Geometry check sheet. Reference: the model listing, model coordinates, mm. Face numbers are marked on the shaded views. Give positions to 0.01 mm unless a question says otherwise; leave off trailing zeros. Loops run counter-clockwise (first coordinate to the right, second up) from the corner with the lowest first, then second, coordinate; pieces in that order, holes last.
1. Release check for a two-part mould opening along Y. For the marked faces 1, 2 and 3 record: +Y half, -Y half, draft (parallel to the pull), parting line (faces both ways), or undercut.
2. Cross-section at A-A, the plane y = -6.5. Record the cut outline in (x, z), plus the area to 3 significant figures.
3. Material ranges on L1, parallel to Z at x = 0, y = -25.5; L2, parallel to Z at x = -4.25, y = 27.5; L3, parallel to X at y = 11, z = -1.5, recorded low to high.
4. Go/stop test with flat-tipped pins: pin 1 Ø1 at (x, z) = (4.5, 0.5) entering from +Y; pin 2 Ø1.5 at (x, y) = (-4, -6.5) entering from -Z; pin 3 Ø2 at (x, y) = (1, -8.5) entering from -Z. Record where each tip stops, or that it passes through.
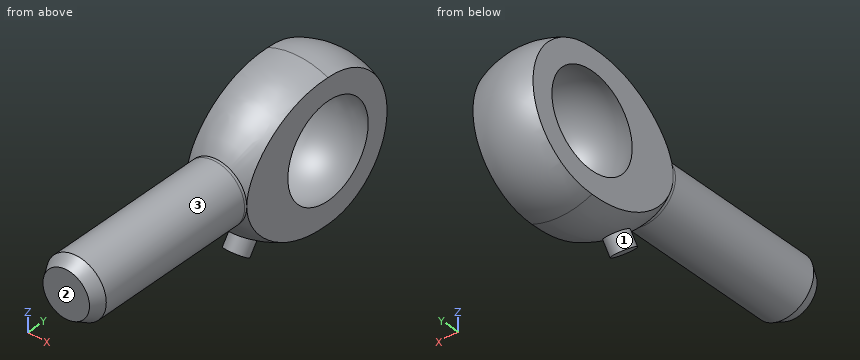
Autodesk Inventor part; units mm, degrees
ref_plane "IP1_XY" through (0, 21, 0) normal (1, 0, 0) x (0, 0, -1)
ref_plane "IP1_YZ" through (0, 21, 0) normal (0, 0, -1) x (0, 1, 0)
ref_plane "IP1_ZX" through (0, 21, 0) normal (0, 1, 0) x (1, 0, 0)
sketch "Sketch_5" plane through (0, 0, 0) normal (0, 0, 1) x (1, 0, 0)
  line L0 (0, -33) -> (0, 36)
  arc A0 (15, 21) -> (0, 36) centre (0, 21) ccw
  arc A1 (6, 2.0892) -> (15, 21) centre (-7.4821, 20.1026) ccw
  arc A2 (6, 2.0892) -> (6, 1.56) centre (8.9883, 1.8246) ccw
  line L1 (6, 1.56) -> (6, -30.66)
  line L2 (6, -30.66) -> (4.649, -33)
  line L3 (4.649, -33) -> (0, -33)
  line L4 (0, -33) -> (0, 36)
revolve "Revolution1" add sketch "Sketch_5" angle 360 about axis through (0, -33, 0) along (0, -1, 0)
thread "Thread1"
sketch "Sketch_6" plane through (0, 0, 0) normal (0, 0, 1) x (1, 0, 0)
  line L0 (-22.5, 37.8) -> (-22.5, -34.65)
  line L1 (-22.5, -34.65) -> (22.5, -34.65)
  line L2 (22.5, -34.65) -> (22.5, 37.8)
  line L3 (22.5, 37.8) -> (-22.5, 37.8)
  line L4 (-6, 36) -> (-6, -33)
  line L5 (-6, -33) -> (6, -33)
  line L6 (6, -33) -> (6, 36)
  line L7 (6, 36) -> (-6, 36)
extrude "Extrusion1" cut sketch "Sketch_6" along normal mid plane 30
sketch "Sketch_7" plane through (0, 0, 0) normal (0, 0, 1) x (1, 0, 0)
  line L0 (11.115, 21) -> (-11.115, 21)
  arc A0 (11.115, 21) -> (-11.115, 21) centre (0, 21) ccw
  line L1 (11.115, 21) -> (-11.115, 21)
revolve "Revolution2" cut sketch "Sketch_7" angle 360 about axis through (11.115, 21, 0) along (1, 0, 0)
sketch "Sketch_14" plane through (0, 0, 0) normal (1, 0, 0) x (0, 1, 0)
  line L0 (6.5961, -13.8934) -> (10.1809, -8.7737)
  line L1 (10.1809, -8.7737) -> (12.024, -10.0643)
  line L2 (12.024, -10.0643) -> (8.4392, -15.184)
  line L3 (8.4392, -15.184) -> (6.5961, -13.8934)
  line L4 (6.5961, -13.8934) -> (10.1809, -8.7737)
revolve "Revolution3" add sketch "Sketch_14" angle 360 about axis through (0, 6.5961, -13.8934) along (0, -0.5735764, -0.819152)
ref_plane "IP1_XY" through (0, 21, 0) normal (1, 0, 0) x (0, 0, -1)
ref_plane "IP1_YZ" through (0, 21, 0) normal (0, 0, -1) x (0, 1, 0)
ref_plane "IP1_ZX" through (0, 21, 0) normal (0, 1, 0) x (1, 0, 0)
properties part number "POS 12 Body"
Result:
1. face 1: undercut
1. face 2: -Y half
1. face 3: draft
2. outline: circle Ø12 at (0, 0)
2. area: 113 mm2
3. L1: z = -6 to 6
3. L2: z = -12.83 to -7.95, 7.95 to 12.83
3. L3: x = -6 to -4.61, 4.61 to 6
4. pin 1: stops at y = 35.45
4. pin 2: stops at z = -5.04
4. pin 3: stops at z = -6
